Verification items for this drawing (mm, ordinates from the low corner). A direction names the side the tool comes from. Coordinates: 2 decimals unless noted, no trailing zeros. Write each loop counter-clockwise with the first axis right and the second up, starting at its lowest first coordinate (ties: lowest second). Pieces come first, ordered by that corner, then holes. Notation, with made-up numbers: (-25, 42) -> (-4, 42) arc R19 ccw to (-4, 53) -> close; hole circle Ø6 at (-21, 68.25). An arc over 180 degrees is marked (long way). One line per item, written item: value. Start each with the question number.
1) Sectioned sample at C-C on x = 73.5. Enter the section's corners in (y, z) (1 decimal).
2) Set-up check for the marked faces 1 and 2: record each of +Z, -Z, +X, -X, +Y, -Y from which the full face is reachable in a straight line by a thin tool's end or side.
3) Sectioned sample at B-B on z = 55. Enter the section's corners in (x, y), plus the area to 3 significant figures.
4) Gauge pin test, flat ends, axial feed: P1, Ø3, axis at y = 53.5, z = 30, coming from the -X side; P2, Ø3.5, axis at x = 77, y = 42, coming from the +Z side (1 decimal); P3, Ø10, axis at x = 75.5, y = 28.5, coming from the -Z side. Record the tip position at first contact, or that the pin passes through.
5) Scan lines: line 1 along X through (y, z) = (4, 37.5); line 2 along X through (y, z) = (45.5, 4.5). Record each from-to range of solid material in increasing order. Write a range as [from, to].
6) Draft check along Z on the marked faces 3, 4, 5 and 6. Enter one of: +Z half, -Z half, draft (parallel to the pull), parting line (faces both ways), or undercut.
7) Sectioned sample at A-A on y = 34.5. Enter the section's corners in (x, z) (1 decimal), plus the area to 3 significant figures.
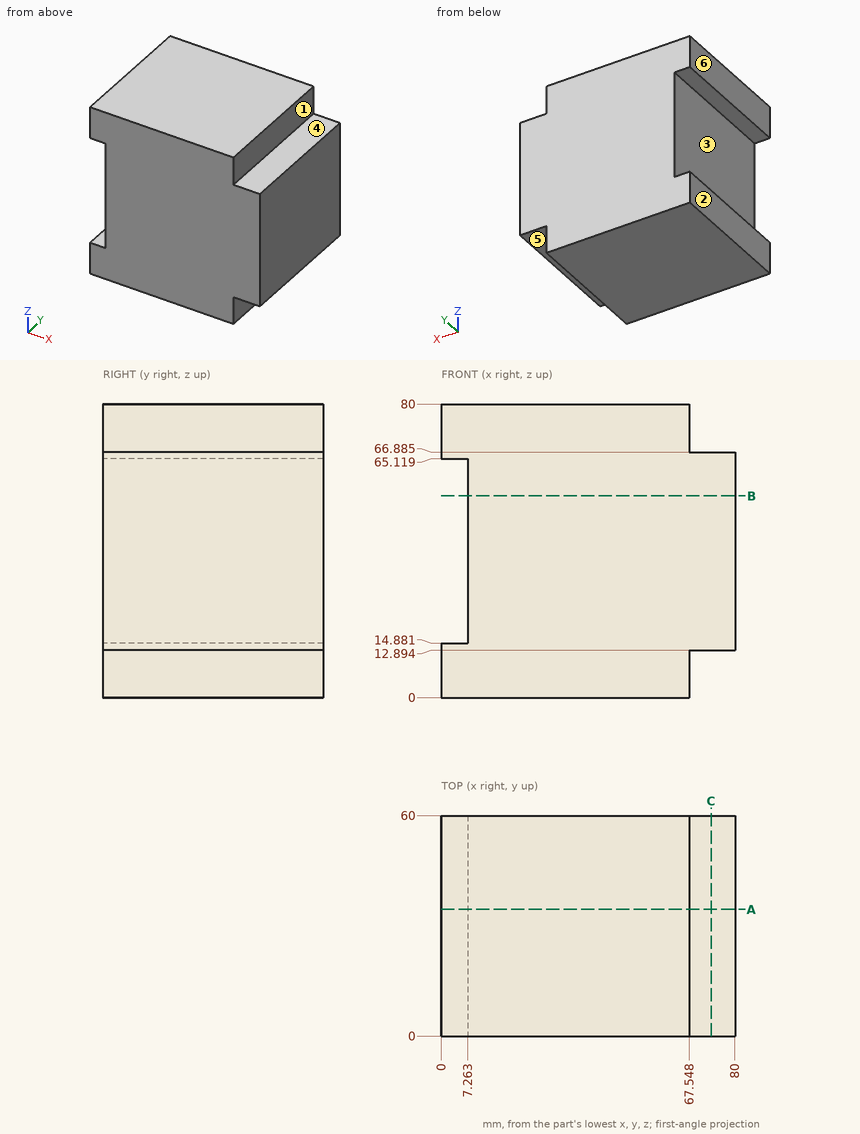
Answers:
1. outline: (0, 12.9) -> (60, 12.9) -> (60, 66.9) -> (0, 66.9) -> close
2. face 1: +Z, +X, +Y, -Y
2. face 2: +Z, -Z, -X, +Y, -Y
3. outline: (7.26, 0) -> (80, 0) -> (80, 60) -> (7.26, 60) -> close
3. area: 4,360 mm2
4. P1: stops at x = 7.26
4. P2: stops at z = 66.9
4. P3: stops at z = 12.89
5. line 1: x = [7.26, 80]
5. line 2: x = [0, 67.55]
6. face 3: undercut
6. face 4: +Z half
6. face 5: -Z half
6. face 6: draft
7. outline: (0, 0) -> (67.5, 0) -> (67.5, 12.9) -> (80, 12.9) -> (80, 66.9) -> (67.5, 66.9) -> (67.5, 80) -> (0, 80) -> (0, 65.1) -> (7.3, 65.1) -> (7.3, 14.9) -> (0, 14.9) -> close
7. area: 5,710 mm2
